Work out the finished part from the listing and answer in its coordinate system (mm). A direction names the side the tool comes from. Give positions to 0.01 mm unless a question says otherwise; leave off trailing zeros. Write each loop counter-clockwise with the first axis right and the second up, starting at its lowest first coordinate (ties: lowest second). Pieces come first, ordered by that corner, then holes. Notation, with made-up numbers: (40.5, 52.5) -> (90.5, 52.5) arc R12 cw to (90.5, 59.5) -> close; hole circle Ø9 at (1, -20). An arc over 180 degrees is marked (long way). Use a Markdown table: item, result. Add a question column.
Q1. Section A-A, the plane x = 3.75 is taken. Give the vertices of the cut face in (y, z), plus the area to 3 significant figures.
Q2. For faces 1 (the face through (3.375, 31, 4)), 2 (the face through (-4.5, 35, -3)), 3 (the face through (-3.375, 30.7, 2)), determine the directions among +Z, -Z, +X, -X, +Y, -Y from which every point of the face is accessible in a straight line to the end or side of a thin tool.
Q3. Each of these flat-tipped pins is pushed along its axis until it touches: pin 1 Ø5 at (x, y) = (-2.5, 29) entering from -Z; pin 2 Ø3 at (x, z) = (0.5, -7.5) entering from -Y; pin 3 Ø2 at (x, y) = (-2.5, 20.5) entering from +Z. Where does it stop, or does it pass through?
Q4. Consider line 1 (X direction, y = 44, z = 1) (3 decimals); line 2 (Y direction, x = 1.8, z = 0); line 3 (Y direction, x = 4, z = 0) (3 decimals). Determine where each line is inside the solid, lowest interval first.
from build123d import *

# Parameters (mm, degrees)
WYTNIJ_WYCI_GNI_CIE1_DEPTH      = 10.998876849
WYTNIJ_WYCI_GNI_CIE1_DEPTH_BACK = 10.998876849
SZKIC4_W                        = 1.45
SZKIC4_H                        = 9
SZKIC8_R                        = 3
WYTNIJ_WYCI_GNI_CIE3_DEPTH      = 5.5
WYTNIJ_WYCI_GNI_CIE3_DEPTH_BACK = 5.5
SKETCH2_W                       = 18.954630749
SKETCH2_H                       = 12.318293367
CUT_EXTRUDE2_DEPTH              = 5.5
CUT_EXTRUDE2_DEPTH_BACK         = 5.5


with BuildPart() as part:
    # Szkic1 one side → Obrót4 (revolve)
    with BuildSketch(Plane.XY):
        with BuildLine():
            Line((-3, 21), (-3, 0))
            Line((-3, 0), (0, 0))
            Line((0, 0), (0.005166955, 46))
            ThreePointArc((0.005166955, 46), (-8.632770826, 41.038455208), (-8.699205566, 31.077206177))
            Line((-8.699205566, 31.077206177), (-3, 21))
        make_face()
    revolve(axis=Axis((0.005166955, 46, 0), (-0.000112325, -0.999999994, 0)))

    # Szkic2 → Wytnij-wyciągnięcie1 (cut, two sides)
    with BuildSketch(Plane.XY) as wytnij_wyci_gni_cie1_sk:
        Polygon((-3.375, 46), (-20, 46), (-20, 10.866665268), (-3.375, 21.663066505), align=None)
        Polygon((20, 46), (3.375, 46), (3.375, 21.65370739), (20, 10.857306153), align=None)
    extrude(amount=WYTNIJ_WYCI_GNI_CIE1_DEPTH, mode=Mode.SUBTRACT)
    extrude(wytnij_wyci_gni_cie1_sk.sketch, amount=-WYTNIJ_WYCI_GNI_CIE1_DEPTH_BACK, mode=Mode.SUBTRACT)

    # Szkic4 → Obrót5 (revolve)
    with BuildSketch(Plane.YX):
        with BuildLine():
            Line((40.449326049, 4.5), (40.449326049, -4.5))
            ThreePointArc((40.449326049, -4.5), (41.839498769, -2.438212993), (42.328030498, 0))
            ThreePointArc((42.328030498, 0), (41.839498769, 2.438212993), (40.449326049, 4.5))
        make_face()
        with Locations((39.724326049, 0)):
            Rectangle(SZKIC4_W, SZKIC4_H)
    revolve(axis=Axis((-0.999999975, 35.999326049, 0), (1, 0, 0)))

    # Szkic8 → Wytnij-wyciągnięcie3 (cut, two sides)
    with BuildSketch(Plane(origin=(0, 0, 0), x_dir=(0, 0, -1), z_dir=(1, 0, 0))) as wytnij_wyci_gni_cie3_sk:
        with Locations((0, 35.999326049)):
            Circle(SZKIC8_R)
    extrude(amount=WYTNIJ_WYCI_GNI_CIE3_DEPTH, mode=Mode.SUBTRACT)
    extrude(wytnij_wyci_gni_cie3_sk.sketch, amount=-WYTNIJ_WYCI_GNI_CIE3_DEPTH_BACK, mode=Mode.SUBTRACT)

    # Sketch2 → Cut-Extrude2 (cut, two sides)
    with BuildSketch(Plane(origin=(0, 0, 0), x_dir=(0, 0, -1), z_dir=(1, 0, 0))) as cut_extrude2_sk:
        with Locations((0.852276563, 4.340516208)):
            Rectangle(SKETCH2_W, SKETCH2_H)
    extrude(amount=CUT_EXTRUDE2_DEPTH, mode=Mode.SUBTRACT)
    extrude(cut_extrude2_sk.sketch, amount=-CUT_EXTRUDE2_DEPTH_BACK, mode=Mode.SUBTRACT)


solid = part.part
Result set:
| question | item | result |
|---|---|---|
| 1 | outline | circle Ø10.2 at (36, 0); hole circle Ø6 at (36, 0) |
| 1 | area | 53.4 mm2 |
| 2 | face 1 | +X |
| 2 | face 2 | +Z, -Z, -X, +Y, -Y |
| 2 | face 3 | -X |
| 3 | pin 1 | stops at z = -8.7 |
| 3 | pin 2 | stops at y = 26.33 |
| 3 | pin 3 | stops at z = 2.6 |
| 4 | line 1 | x = -3.375 to 3.375 |
| 4 | line 2 | y = 10.5 to 33, 39 to 45.84 |
| 4 | line 3 | y = 31.095 to 32.999, 38.999 to 40.904 |
